Model file for the job. Use its own axes, mm. Give positions to 0.01 mm unless a question says otherwise; leave off trailing zeros. Order: outer loops, then holes, each group sorted by start corner. A loop starts at its lowest first (then second) coordinate and runs counter-clockwise, first axis right, second up. Notation, with made-up numbers: (55.25, -31) -> (102.25, -31) arc R23 cw to (102.25, -3) -> close; hole circle Ø10 at (-30.75, 68). An arc over 180 degrees is marked (long way). Use CSV: the item, a comma, the result in double quotes. Start each with the question number.
1. Drop flat-ended pins along their axis: pin 1 (1 mm diameter, centred on x = -15.5, y = -3.5, fed in from -Z); pin 2 (12 mm diameter, centred on x = 16.5, y = -4.5, fed in from +Z). Give the stop position or say it passes through.
2. Cut at A-A on y = 0. List the corners of the cut face in (x, z), then the cut area to 3 significant figures.
3. Cut at C-C on x = 18. List the corners of the cut face in (y, z), then the cut area to 3 significant figures.
4. Wall check: line 1 (X direction, y = -3, z = 1.2); line 2 (Y direction, x = -7.5, z = 1.05); line 3 (X direction, y = 1, z = 1.25). Give the ranges that are in metal, low to high. Write a range as from..to.
5. Pull direction Y, two halves, no side cores. Call faces 1 (the cylindrical face through (10.64, 11.04, 0.78)), 2 (the cylindrical face through (-0.1, 15.08, 0.8)), 3 (the flat face through (10, -10, 1.588)), 4 (the cylindrical face through (-18.267, -14.007, 0.783)): released by +Y, released by -Y, zero draft, split by the parting line, or undercut.
6. Cut at D-D on z = 0.8. Give the number of separate pieces and of enclosed holes in the cut face, then the cut area to 3 significant figures.
```python
from build123d import *

# Parameters (mm, degrees)
F0_R            = 23.01875
F0_R_2          = 2.15265
F0_R_3          = 11.90625
F1_DEPTH        = 1.5875
F3_DEPTH        = 1.5875
F3_COPIES_COUNT = 4


# Not quite as in the source:
# - a pattern or mirror of a feature is missing from the dataset's text; its kind, count and spacing are read off the source's solid


with BuildPart() as f1:
    # F0 (on Top) → F1 (new body)
    with BuildSketch(Plane.XY):
        Circle(F0_R)
        with Locations((-12.3478521665, -12.3478521665)):
            Circle(F0_R_2, mode=Mode.SUBTRACT)
        with Locations((12.3478521665, -12.3478521665)):
            Circle(F0_R_2, mode=Mode.SUBTRACT)
        with Locations((-12.3478521665, 12.3478521665)):
            Circle(F0_R_2, mode=Mode.SUBTRACT)
        Circle(F0_R_3, mode=Mode.SUBTRACT)
        with Locations((12.3478521665, 12.3478521665)):
            Circle(F0_R_2, mode=Mode.SUBTRACT)
    extrude(amount=F1_DEPTH)

    # F2 (on face) → F3 (cut, through all)
    with BuildSketch(Plane.XY.offset(1.5875)):
        with BuildLine():
            ThreePointArc((-9.7719120136, 17.2709047146), (-7.8938999882, 15.6696324205), (-6.8946489019, 13.4129757356))
            ThreePointArc((-6.8946489019, 13.4129757356), (0, 15.08125), (6.8946489019, 13.4129757356))
            ThreePointArc((6.8946489019, 13.4129757356), (7.8938999882, 15.6696324205), (9.7719120136, 17.2709047146))
            ThreePointArc((9.7719120136, 17.2709047146), (0, 19.84375), (-9.7719120136, 17.2709047146))
        make_face()
    f3 = extrude(amount=-F3_DEPTH, mode=Mode.SUBTRACT)

    # F3_copies: F3 ×4 about axis
    f3_copies_axis = Axis((0, 0, 0), (0, 0, 1))
    for i in range(1, F3_COPIES_COUNT):
        add(f3.rotate(f3_copies_axis, i * 360 / F3_COPIES_COUNT), mode=Mode.SUBTRACT)


solid = f1.part
```
Verdict:
1,pin 1,"through"
1,pin 2,"z = 1.59"
2,outline,"(-23.02, 0) -> (-19.84, 0) -> (-19.84, 1.59) -> (-23.02, 1.59) -> close; (-15.08, 0) -> (-11.91, 0) -> (-11.91, 1.59) -> (-15.08, 1.59) -> close; (11.91, 0) -> (15.08, 0) -> (15.08, 1.59) -> (11.91, 1.59) -> close; (19.84, 0) -> (23.02, 0) -> (23.02, 1.59) -> (19.84, 1.59) -> close"
2,area,"20.2 mm^2"
3,outline,"(-14.35, 0) -> (-8.35, 0) -> (-8.35, 1.59) -> (-14.35, 1.59) -> close; (8.35, 0) -> (14.35, 0) -> (14.35, 1.59) -> (8.35, 1.59) -> close"
3,area,"19.0 mm^2"
4,line 1,"-22.82..-19.62, -14.78..-11.52, 11.52..14.78, 19.62..22.82"
4,line 2,"-21.76..-18.37, -15.06..-9.25, 9.25..15.06, 18.37..21.76"
4,line 3,"-23..-19.82, -15.05..-11.86, 11.86..15.05, 19.82..23"
5,face 1,"undercut"
5,face 2,"undercut"
5,face 3,"zero draft"
5,face 4,"split by the parting line"
6,separate pieces,"1"
6,enclosed holes,"9"
6,area,"844 mm^2"
